from build123d import *

# Parameters (mm, degrees)
F1_DEPTH = 24.495
F1_TAPER = 19.4657
F2_SIZE  = 1


with BuildPart() as f1:
    # F0 (on Top) → F1 (new body)
    with BuildSketch(Plane.XY):
        Polygon((15, 8.6602540378), (-15, 8.6602540378), (0, -17.3205080757), align=None)
    extrude(amount=F1_DEPTH, taper=F1_TAPER)

    # F2 (call 1 of 3: OpenCascade refuses the feature's edges together)
    f2_edges = [f1.edges().sort_by_distance(p)[0] for p in [
        (0, -8.662872, 12.247501),
    ]]
    chamfer(f2_edges, length=F2_SIZE)

    # F2#2 (call 2 of 3)
    f2_2_edges = [f1.edges().sort_by_distance(p)[0] for p in [
        (7.502267, 4.331436, 12.247501),
    ]]
    chamfer(f2_2_edges, length=F2_SIZE)

    # F2#3 (call 3 of 3)
    f2_3_edges = [f1.edges().sort_by_distance(p)[0] for p in [
        (-7.502267, 4.331436, 12.247501),
    ]]
    chamfer(f2_3_edges, length=F2_SIZE)


solid = f1.part
For this review, take the finished solid that the model builds, in its own axes (mm). Give positions to 0.01 mm unless a question says otherwise; leave off trailing zeros. Order: outer loops, then holes, each group sorted by start corner. A loop starts at its lowest first (then second) coordinate and runs counter-clockwise, first axis right, second up. Notation, with made-up numbers: M 1.5,55 L 30.5,55 A17 cw 30.5,74 Z; hole C -34,73 d6. An arc over 180 degrees is marked long. Answer in a Markdown table with one row per item. Add a question column.
(1) Consider section B-B on z = 15.25. State the section outline as (x, y) points, and give its area (3 significant figures).
(2) Consider section A-A on y = 4. State the section outline as (x, z) points, and give its area (3 significant figures).
(3) Consider section D-D on y = -3.75. State the section outline as (x, z) points, and give its area (3 significant figures).
(4) Wall thickness on probe 1 along X at (y, z) = (0, 8.25); probe 2 along Y at (x, z) = (-4, 4.5); probe 3 along Z at (x, y) = (-4.25, -9.5): over which ranges is each line inside the solid? List them lowest first. Write a range as [from, to].
(5) For pin 1 (10 mm diameter, centred on x = -4, y = 3.5, fed in from +Z); pin 2 (8 mm diameter, centred on y = 2, z = 17.5, fed in from -X); pin 3 (8 mm diameter, centred on x = 1.5, z = 13.5, fed in from -Y), all flat-tipped, find the tip position at first contact; note any pin that passes through.
(6) Consider section C-C on x = 1.25. State the section outline as (y, z) points, and give its area (3 significant figures).
Evaluation:
| question | item | result |
|---|---|---|
| 1 | outline | M -5.09,2.27 L -0.58,-5.54 L 0.58,-5.54 L 5.09,2.27 L 4.51,3.27 L -4.51,3.27 Z |
| 1 | area | 53.8 mm^2 |
| 2 | outline | M -12.31,0 L 12.31,0 L 8.08,10.36 L 5.77,13.19 L -5.77,13.19 L -8.08,10.36 Z |
| 2 | area | 250 mm^2 |
| 3 | outline | M -7.83,0 L 7.83,0 L 0.58,17.78 L -0.58,17.78 Z |
| 3 | area | 150 mm^2 |
| 4 | probe 1 | x = [-6.63, 6.63] |
| 4 | probe 2 | y = [-7.21, 7.07] |
| 4 | probe 3 | z = [0, 0.65] |
| 5 | pin 1 | stops at z = 22.73 |
| 5 | pin 2 | stops at x = -6.1 |
| 5 | pin 3 | stops at y = -9.53 |
| 6 | outline | M -15.16,0 L 8.66,0 L 1.39,20.57 L 0.06,21.52 Z |
| 6 | area | 267 mm^2 |
